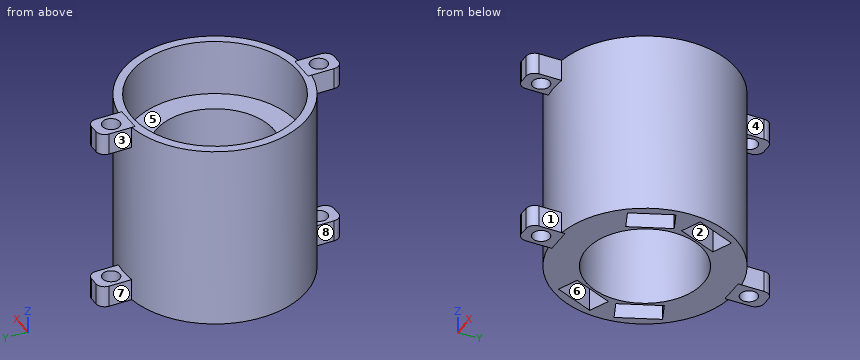
```python
from build123d import *

# Parameters (mm, degrees)
SKETCH1_R                = 19.01
SKETCH1_R_2              = 13.5
BOSS_EXTRUDE1_DEPTH      = 30
BOSS_EXTRUDE2_DEPTH      = 13
BOSS_EXTRUDE2_DEPTH_BACK = 30
SKETCH2_R                = 21
SKETCH2_R_2              = 19.01
CUT_EXTRUDE1_DEPTH       = 28
MIRROR2_COPY_1_DEPTH     = 28
BOSS_EXTRUDE3_START      = -5
SKETCH4_W                = 6
SKETCH4_H                = 8
SKETCH4_R                = 2
BOSS_EXTRUDE3_DEPTH      = 5.0001
FILLET1_R                = 2
FILLET1_OF_MIRROR5_R     = 2
BOSS_EXTRUDE6_START      = 0.0001
SKETCH7_W                = 6
SKETCH7_H                = 8
SKETCH7_R                = 2
BOSS_EXTRUDE6_DEPTH      = 5.0001
FILLET2_R                = 2


with BuildPart() as part:
    # Sketch1 → Boss-Extrude1 (new body)
    with BuildSketch(Plane.XY):
        Circle(SKETCH1_R)
        Circle(SKETCH1_R_2, mode=Mode.SUBTRACT)
    extrude(amount=BOSS_EXTRUDE1_DEPTH)

    # Sketch2 → Boss-Extrude2 (add, two sides: drawn at the far end of the back side and taken through both)
    with BuildSketch(Plane.XY.offset(30).offset(-BOSS_EXTRUDE2_DEPTH_BACK)):
        Circle(SKETCH2_R)
        Circle(SKETCH2_R_2, mode=Mode.SUBTRACT)
    extrude(amount=BOSS_EXTRUDE2_DEPTH + BOSS_EXTRUDE2_DEPTH_BACK)

    # Sketch3 → Cut-Extrude1 (cut)
    with BuildSketch(Plane(origin=(0, 0, 0), x_dir=(-1, 0, 0), z_dir=(0, 0, -1))):
        Polygon((15.540276616, 12.01617991), (10.937752349, 10.062524267), (14.845063634, 0.857475733), (19.447587901, 2.811131375), align=None)
    cut_extrude1 = extrude(amount=-CUT_EXTRUDE1_DEPTH, mode=Mode.SUBTRACT)

    # Mirror1: Cut-Extrude1 across plane
    add(cut_extrude1.mirror(Plane.ZX), mode=Mode.SUBTRACT)

    # Mirror2: Cut-Extrude1 across plane
    add(cut_extrude1.mirror(Plane(origin=(0, 0, 0), x_dir=(0, 0, 1), z_dir=(1, 0, 0))), mode=Mode.SUBTRACT)

    # Mirror2 copy 1 sketch → Mirror2 copy 1 (cut)
    with BuildSketch(Plane(origin=(0, 0, 0), x_dir=(1, 0, 0), z_dir=(0, 0, -1))):
        Polygon((15.540276616, 12.01617991), (10.937752349, 10.062524267), (14.845063634, 0.857475733), (19.447587901, 2.811131375), align=None)
    extrude(amount=-MIRROR2_COPY_1_DEPTH, mode=Mode.SUBTRACT)

    # Sketch4 → Boss-Extrude3 (add)
    with BuildSketch(Plane(origin=(0, 0, 0), x_dir=(-1, 0, 0), z_dir=(0, 0, -1)).offset(BOSS_EXTRUDE3_START)):
        with Locations((0, 24)):
            Rectangle(SKETCH4_W, SKETCH4_H)
        with Locations((0, 24)):
            Circle(SKETCH4_R, mode=Mode.SUBTRACT)
    boss_extrude3 = extrude(amount=BOSS_EXTRUDE3_DEPTH)

    # Fillet1
    fillet1_edges = [part.edges().sort_by_distance(p)[0] for p in [
        (-3, 28, 2.49995),
        (3, 28, 2.49995),
    ]]
    fillet(fillet1_edges, radius=FILLET1_R)

    # Mirror5: Boss-Extrude3 across plane
    add(boss_extrude3.mirror(Plane.ZX))

    # Fillet1 of Mirror5
    fillet1_of_mirror5_edges = [part.edges().sort_by_distance(p)[0] for p in [
        (-3, -28, 2.49995),
        (3, -28, 2.49995),
    ]]
    fillet(fillet1_of_mirror5_edges, radius=FILLET1_OF_MIRROR5_R)

    # Sketch7 → Boss-Extrude6 (add)
    with BuildSketch(Plane.XY.offset(43).offset(BOSS_EXTRUDE6_START)):
        with Locations((0, 24)):
            Rectangle(SKETCH7_W, SKETCH7_H)
        with Locations(Location((0, 24, 0), (0, 0, 180))):
            Circle(SKETCH7_R, mode=Mode.SUBTRACT)
    boss_extrude6 = extrude(amount=-BOSS_EXTRUDE6_DEPTH)

    # Mirror6: Boss-Extrude6 across plane
    add(boss_extrude6.mirror(Plane.ZX))

    # Fillet2
    fillet2_edges = [part.edges().sort_by_distance(p)[0] for p in [
        (-3, 28, 40.50005),
        (3, 28, 40.50005),
        (-3, -28, 40.50005),
        (3, -28, 40.50005),
    ]]
    fillet(fillet2_edges, radius=FILLET2_R)


solid = part.part
```
For this review, take the finished solid that the model builds, in its own axes (mm). Face numbers are marked on the shaded views. A direction names the side the tool comes from. Round coordinates to 2 decimals unless told otherwise and drop trailing zeros. Order: outer loops, then holes, each group sorted by start corner. A loop starts at its lowest first (then second) coordinate and runs counter-clockwise, first axis right, second up.
Q1. Mouldability with a two-part tool opening along X and no side actions: class the marked faces 1, 2 and 3 as pulls with the +X half, pulls with the -X half, needs draft (parallel to the pull), parting line crosses it, or undercut.
Findings below:
face 1: pulls with the +X half
face 2: undercut
face 3: pulls with the -X half
Q2. We need section C-C, the plane y = -2. Give the boundary of the cut face in (x, z).
Findings below:
outline: (-20.9, 0) - (-17.54, 0) - (-17.54, 28) - (-14.36, 28) - (-14.36, 0) - (-13.35, 0) - (-13.35, 30) - (-18.9, 30) - (-18.9, 43) - (-20.9, 43) - close; (13.35, 0) - (14.36, 0) - (14.36, 28) - (17.54, 28) - (17.54, 0) - (20.9, 0) - (20.9, 43) - (18.9, 43) - (18.9, 30) - (13.35, 30) - close
Q3. Machinability: for the marked faces 4, 5, 6, 7 and 8, which of the approach directions +Z, -Z, +X, -X, +Y, -Y give a long, thin tool a straight path to every point of the face, cutting with its end or side? Answer none if there is none.
Findings below:
face 4: +Z, -Z, +X, +Y
face 5: +Z
face 6: -Z
face 7: +Z, -Z, -X, +Y
face 8: +Z, -Z, -X, -Y
Q4. We need section D-D, the plane x = -12. Give the boundary of the cut face in (y, z), plus the area to 3 significant figures.
Findings below:
outline: (-17.23, 0) - (-10.51, 0) - (-10.51, 28) - (-7.56, 28) - (-7.56, 0) - (-6.18, 0) - (-6.18, 30) - (-14.74, 30) - (-14.74, 43) - (-17.23, 43) - close; (6.18, 0) - (7.56, 0) - (7.56, 28) - (10.51, 28) - (10.51, 0) - (17.23, 0) - (17.23, 43) - (14.74, 43) - (14.74, 30) - (6.18, 30) - close
area: 562 mm2
Q5. Insertion check: P1, Ø8, axis at x = -8.5, z = 17.5, coming from the +Y side; P2, Ø10, axis at y = -9, z = 20, coming from the +X side; P3, Ø5, axis at x = 2, z = 25, coming from the +Y side; P4, Ø2.5, axis at x = 0, y = -24, coming from the -Z side. Each pin has a flat end and moves straight along its axis. Give the tip position at first contact, or say it passes through.
Findings below:
P1: stops at y = 20.51
P2: stops at x = 20.62
P3: stops at y = 21
P4: passes through
Q6. Wall thickness on line 1 (X direction, y = 24, z = 39.95); line 2 (Z direction, x = -2.5, y = -21); line 3 (Y direction, x = -11.5, z = 11): over which ranges is each line inside the solid? List them lowest first.
Findings below:
line 1: x = -3 to -2, 2 to 3
line 2: z = 0 to 5, 38 to 43
line 3: y = -17.57 to -10.3, -8.74 to -7.07, 7.07 to 8.74, 10.3 to 17.57
Q7. We need section B-B, the plane z = 10. Give the boundary of the cut face in (x, y).
Findings below:
outline: circle Ø42 at (0, 0); hole (-19.45, -2.81) - (-15.54, -12.02) - (-10.94, -10.06) - (-14.85, -0.86) - close; hole (-19.45, 2.81) - (-14.85, 0.86) - (-10.94, 10.06) - (-15.54, 12.02) - close; hole circle Ø27 at (0, 0); hole (10.94, -10.06) - (15.54, -12.02) - (19.45, -2.81) - (14.85, -0.86) - close; hole (10.94, 10.06) - (14.85, 0.86) - (19.45, 2.81) - (15.54, 12.02) - close
Q8. We need section A-A, the plane y = -24. Give the boundary of the cut face in (x, z), plus the area to 3 significant figures.
Findings below:
outline: (-3, 0) - (-2, 0) - (-2, 5) - (-3, 5) - close; (-3, 38) - (-2, 38) - (-2, 43) - (-3, 43) - close; (2, 0) - (3, 0) - (3, 5) - (2, 5) - close; (2, 38) - (3, 38) - (3, 43) - (2, 43) - close
area: 20.0 mm2
